Geometry check sheet. Reference: the model listing, model coordinates, mm. A direction names the side the tool comes from. Coordinates: 2 decimals unless noted, no trailing zeros. Loops run counter-clockwise (first coordinate to the right, second up) from the corner with the lowest first, then second, coordinate; pieces in that order, holes last. Notation, with made-up numbers: (22.25, -1) - (32.25, -1) arc R34 ccw to (32.25, 34) - close; hole circle Ø4 at (23, 85). An arc over 180 degrees is marked (long way). One line per item, written item: value.
from build123d import *

# Parameters (mm, degrees)
BOSS_EXTRUDE1_DEPTH            = 25
CUT_EXTRUDE1_DEPTH             = 5
CUT_EXTRUDE7_REACH             = 136.629
CUT_EXTRUDE7_DIRECTION_2_REACH = 136.629
CUT_EXTRUDE8_REACH             = 136.629
CUT_EXTRUDE8_DIRECTION_2_REACH = 136.629
CUT_EXTRUDE9_DEPTH             = 40
CUT_EXTRUDE9_DEPTH_BACK        = 40
FILLET2_R                      = 15
BOSS_EXTRUDE5_DEPTH            = 17
FILLET3_R                      = 5


with BuildPart() as part:
    # Sketch1 → Boss-Extrude1 (new body)
    with BuildSketch(Plane(origin=(0, 0, 0), x_dir=(1, 0, 0), z_dir=(0, 1, 0))):
        Polygon((0, 0), (-50, 86.6025403784439), (-149.99999999999997, 86.60254037844393), (-199.99999999999997, 1.041e-14), (-150.00000000000003, -86.60254037844386), (-50.00000000000001, -86.60254037844389), align=None)
    extrude(amount=BOSS_EXTRUDE1_DEPTH)

    # Sketch6 → Cut-Extrude1 (cut)
    with BuildSketch(Plane(origin=(0, 25, 0), x_dir=(1, 0, 0), z_dir=(0, 1, 0))):
        Polygon((-180, 5.476e-14), (-139.99999999999997, -69.28203230275507), (-59.99999999999997, -69.28203230275508), (-20.000000000000004, 1.463e-14), (-60.000000000000014, 69.28203230275516), (-140, 69.28203230275516), align=None)
    extrude(amount=-CUT_EXTRUDE1_DEPTH, mode=Mode.SUBTRACT)

    # Cut-Extrude7: up to this plane
    cut_extrude7_end = Plane(origin=(-20.000000000000004, 20, -1.463e-14), z_dir=(0.8660254037844388, 0, -0.49999999999999983))
    # Sketch21 → Cut-Extrude7 (cut, up to the surface)
    with BuildSketch(Plane(origin=(-100, 0, 0), x_dir=(0, 0, -1), z_dir=(1, 0, 0)), mode=Mode.PRIVATE) as cut_extrude7_sk1:
        Polygon((69.28203230275516, 20), (69.28203230275516, 10.263045350293245), (3.123e-14, 20), align=None)
    cut_extrude7_tool1 = split(extrude(cut_extrude7_sk1.sketch, amount=CUT_EXTRUDE7_REACH, mode=Mode.PRIVATE), bisect_by=cut_extrude7_end, keep=Keep.BOTH, mode=Mode.PRIVATE)
    add(cut_extrude7_tool1.solids().sort_by_distance((-100, 16.754348, -46.188022))[0], mode=Mode.SUBTRACT)

    # Cut-Extrude7 direction 2: up to this plane
    cut_extrude7_direction_2_end = Plane(origin=(-140, 20, -69.28203230275516), z_dir=(-0.8660254037844388, 0, -0.4999999999999998))
    # Sketch21 → Cut-Extrude7 direction 2 (cut, up to the surface)
    with BuildSketch(Plane(origin=(-100, 0, 0), x_dir=(0, 0, -1), z_dir=(1, 0, 0)), mode=Mode.PRIVATE) as cut_extrude7_direction_2_sk1:
        Polygon((69.28203230275516, 20), (69.28203230275516, 10.263045350293245), (3.123e-14, 20), align=None)
    cut_extrude7_direction_2_tool1 = split(extrude(cut_extrude7_direction_2_sk1.sketch, amount=-CUT_EXTRUDE7_DIRECTION_2_REACH, mode=Mode.PRIVATE), bisect_by=cut_extrude7_direction_2_end, keep=Keep.BOTH, mode=Mode.PRIVATE)
    add(cut_extrude7_direction_2_tool1.solids().sort_by_distance((-100, 16.754348, -46.188022))[0], mode=Mode.SUBTRACT)

    # Cut-Extrude8: up to this plane
    cut_extrude8_end = Plane(origin=(-59.99999999999997, 20, 69.28203230275508), z_dir=(0.8660254037844388, 0, 0.49999999999999967))
    # Sketch22 → Cut-Extrude8 (cut, up to the surface)
    with BuildSketch(Plane(origin=(-100, 0, 0), x_dir=(0, 0, -1), z_dir=(1, 0, 0)), mode=Mode.PRIVATE) as cut_extrude8_sk1:
        Polygon((3.123e-14, 20), (-69.28203230275508, 10.26304535029323), (-69.28203230275508, 20), align=None)
    cut_extrude8_tool1 = split(extrude(cut_extrude8_sk1.sketch, amount=CUT_EXTRUDE8_REACH, mode=Mode.PRIVATE), bisect_by=cut_extrude8_end, keep=Keep.BOTH, mode=Mode.PRIVATE)
    add(cut_extrude8_tool1.solids().sort_by_distance((-100, 16.754348, 46.188022))[0], mode=Mode.SUBTRACT)

    # Cut-Extrude8 direction 2: up to this plane
    cut_extrude8_direction_2_end = Plane(origin=(-180, 20, -5.476e-14), z_dir=(-0.8660254037844387, 0, 0.5))
    # Sketch22 → Cut-Extrude8 direction 2 (cut, up to the surface)
    with BuildSketch(Plane(origin=(-100, 0, 0), x_dir=(0, 0, -1), z_dir=(1, 0, 0)), mode=Mode.PRIVATE) as cut_extrude8_direction_2_sk1:
        Polygon((3.123e-14, 20), (-69.28203230275508, 10.26304535029323), (-69.28203230275508, 20), align=None)
    cut_extrude8_direction_2_tool1 = split(extrude(cut_extrude8_direction_2_sk1.sketch, amount=-CUT_EXTRUDE8_DIRECTION_2_REACH, mode=Mode.PRIVATE), bisect_by=cut_extrude8_direction_2_end, keep=Keep.BOTH, mode=Mode.PRIVATE)
    add(cut_extrude8_direction_2_tool1.solids().sort_by_distance((-100, 16.754348, 46.188022))[0], mode=Mode.SUBTRACT)

    # Sketch23 → Cut-Extrude9 (cut, two sides: drawn at the far end of the back side and taken through both)
    with BuildSketch(Plane(origin=(-100, 0, 0), x_dir=(0, 0, -1), z_dir=(1, 0, 0)).offset(-CUT_EXTRUDE9_DEPTH_BACK)):
        Polygon((69.28203230275516, 10.263045350293245), (89.28203230275517, 7.452228656245558), (89.28203230275517, 12.501366518838644), (69.28203230275516, 15.312183212886326), align=None)
        Polygon((-69.28203230275516, 15.312183212886326), (-69.28203230275516, 10.263045350293245), (-89.28203230275517, 7.452228656245558), (-89.28203230275517, 12.501366518838644), align=None)
    extrude(amount=CUT_EXTRUDE9_DEPTH + CUT_EXTRUDE9_DEPTH_BACK, mode=Mode.SUBTRACT)

    # Fillet2
    fillet2_edges = [part.edges().sort_by_distance(p)[0] for p in [
        (-100, 20, -3.347e-14),
    ]]
    fillet(fillet2_edges, radius=FILLET2_R)

    # Sketch27 → Boss-Extrude5 (add)
    # profile 1 of 2: a face of its own
    with BuildSketch(Plane(origin=(0, 25, 0), x_dir=(1, 0, 0), z_dir=(0, 1, 0))):
        Polygon((-147.1132486552964, -81.60254038059946), (-52.8867513447036, -81.60254038059949), (-5.773502689407191, -2.776e-14), (-52.88675134470361, 81.60254038059944), (-147.1132486552964, 81.60254038059945), (-194.22649731059275, -2.775e-14), align=None)
        Polygon((-54.42264973081038, -78.94228634059947), (-8.845299461620776, -2.374e-14), (-54.4226497308104, 78.9422863405995), (-145.57735026918957, 78.9422863405995), (-191.1547005383792, -1.365e-14), (-145.57735026918962, -78.94228634059945), align=None, mode=Mode.SUBTRACT)
    # profile 2 of 2: a face of its own
    with BuildSketch(Plane(origin=(0, 25, 0), x_dir=(1, 0, 0), z_dir=(0, 1, 0))):
        Polygon((-141.5358983848622, -71.94228634059951), (-58.46410161513772, -71.94228634059952), (-16.92820323027549, 1.392e-14), (-58.4641016151377, 71.94228634059947), (-141.53589838486224, 71.94228634059947), (-183.0717967697245, -2.773e-14), align=None)
        Polygon((-139.99999999999997, -69.28203230275507), (-180, 6.939e-14), (-140, 69.28203230275516), (-60.000000000000014, 69.28203230275516), (-20.000000000000004, 1.463e-14), (-59.99999999999997, -69.28203230275508), align=None, mode=Mode.SUBTRACT)
    extrude(amount=BOSS_EXTRUDE5_DEPTH)

    # Fillet3
    fillet3_edges = [part.edges().sort_by_distance(p)[0] for p in [
        (-50.00000000000001, 12.5, 86.60254037844389),
        (-150.00000000000003, 12.5, 86.60254037844386),
        (-147.1132486552964, 33.5, 81.60254038059946),
        (-199.99999999999997, 12.5, -1.041e-14),
        (-52.8867513447036, 33.5, 81.60254038059949),
        (-5.773502689407191, 33.5, 2.776e-14),
        (-149.99999999999997, 12.5, -86.60254037844393),
        (-52.88675134470361, 33.5, -81.60254038059944),
        (-147.1132486552964, 33.5, -81.60254038059945),
        (-50, 12.5, -86.6025403784439),
        (0, 12.5, 0),
        (-191.1547005383792, 33.5, 1.365e-14),
    ]]
    fillet(fillet3_edges, radius=FILLET3_R)


solid = part.part
(1) Cross-section at B-B on x = -105. Record the cut outline in (y, z).
Reply:
outline: (0, -86.6) - (7.83, -86.6) - (19.71, -2.09) arc R15 ccw to (19.71, 2.09) - (7.83, 86.6) - (0, 86.6) - close; (12.88, -86.6) - (25, -86.6) - (25, -81.6) - (42, -81.6) - (42, -78.94) - (25, -78.94) - (25, -71.94) - (42, -71.94) - (42, -69.28) - (15.31, -69.28) - close; (12.88, 86.6) - (15.31, 69.28) - (42, 69.28) - (42, 71.94) - (25, 71.94) - (25, 78.94) - (42, 78.94) - (42, 81.6) - (25, 81.6) - (25, 86.6) - close
(2) Cross-section at C-C on z = -56. Record the cut outline in (x, y).
Reply:
outline: (-167.67, 0) - (-32.33, 0) - (-32.33, 25) - (-38.11, 25) - (-38.11, 42) - (-41.18, 42) - (-41.18, 25) - (-49.26, 25) - (-49.26, 42) - (-52.33, 42) - (-52.33, 12.13) - (-147.67, 12.13) - (-147.67, 42) - (-150.74, 42) - (-150.74, 25) - (-158.82, 25) - (-158.82, 42) - (-161.89, 42) - (-161.89, 25) - (-167.67, 25) - close
(3) Cross-section at A-A on y = 37. State how many separate pieces and enclosed holes the cut face has, and give its area (3 significant figures).
Reply:
separate pieces: 2
enclosed holes: 2
area: 2,780 mm2
(4) Cross-section at D-D on x = -162.5. Record the cut outline in (y, z), and give its area (3 significant figures).
Reply:
outline: (0, -64.95) - (25, -64.95) - (25, -54.95) - (42, -54.95) - (42, -49.63) - (25, -49.63) - (25, -35.63) - (42, -35.63) - (42, -30.31) - (15.74, -30.31) - (19.71, -2.09) arc R15 ccw to (19.71, 2.09) - (15.74, 30.31) - (42, 30.31) - (42, 35.63) - (25, 35.63) - (25, 49.63) - (42, 49.63) - (42, 54.95) - (25, 54.95) - (25, 64.95) - (0, 64.95) - close
area: 3,180 mm2
(5) Go/stop test with flat-tipped pins: pin 1 Ø8.5 at (x, y) = (-111, 34.5) entering from -Z; pin 2 Ø8.5 at (x, y) = (-84.5, 34.5) entering from +Z; pin 3 Ø1.5 at (x, z) = (-107, -41) entering from +Y. Record where each tip stops, or that it passes through.
Reply:
pin 1: z = -81.6
pin 2: z = 81.6
pin 3: y = 14.34
(6) Release check for a two-part mould opening along Z. For faces 1 (the face through (-101.1, 15.17, 34.36)), 2 (the face through (-101, 0, -1)), 3 (the face through (-50.355, 12.675, -85.914)) record: pulls with the +Z half, pulls with the -Z half, needs draft (parallel to the pull), parting line crosses it, or undercut.
Reply:
face 1: undercut
face 2: needs draft
face 3: pulls with the -Z half
(7) Material ranges on probe 1 along Z at (x, y) = (-107, 29); probe 2 along Z at (x, y) = (-126.5, 22); probe 3 along Z at (x, y) = (-175, 27), recorded low to high. Write a range as from..to.
Reply:
probe 1: -81.6..-78.94, -71.94..-69.28, 69.28..71.94, 78.94..81.6
probe 2: -86.6..-69.28, 69.28..86.6
probe 3: -33.3..-27.98, -13.98..-8.66, 8.66..13.98, 27.98..33.3
(8) Access from +Z, -Z, +X, -X, +Y, -Y to the whole of each face (thin tool, end or side, straight path). Record for faces 4 (the face through (-29.64, 33.38, 41.34)), 5 (the face through (-140, 12, -78)), 6 (the face through (-167.95, 33.38, 40.19)), 7 (the face through (-101, 33, 81.603)).
Reply:
face 4: +Z, +X, +Y
face 5: none
face 6: +Y
face 7: +Z, +X, -X, +Y
